Could you check a few things on this model? Use its own coordinates, in mm. Round coordinates to 2 decimals unless told otherwise and drop trailing zeros. Loops run counter-clockwise (first coordinate to the right, second up) from the corner with the lowest first, then second, coordinate; pieces in that order, holes last. Notation, with made-up numbers: (7, -15) -> (14, -15) arc R20 cw to (14, -4) -> close; hole circle Ø6 at (62, 31). An arc over 180 degrees is marked (long way). Write each question's results on one line, items separated by ' | '.
from build123d import *

# Parameters (mm, degrees)
F0_R     = 12.7
F1_DEPTH = 63.5
F2_SIZE  = 5.08


# Not quite as in the source:
# - a fillet or chamfer that OpenCascade refuses, or shapes differently, is made with other operations: its cross-section is extruded or revolved along the edge and cut away or added


with BuildPart() as f1:
    # F0 (on Front) → F1 (new body)
    with BuildSketch(Plane.XZ):
        Circle(F0_R)
    extrude(amount=F1_DEPTH)

    # F2
    f2_edges = [f1.edges().sort_by_distance(p)[0] for p in [
        (-12.7, 0, 0),
    ]]
    chamfer(f2_edges, length=F2_SIZE)

    # F3: fillet of radius 12.7 on 1 edges, made by hand

    # F3_s1 → F3_t2 (revolve, cut)
    with BuildSketch(Plane.XY):
        with BuildLine():
            add(Edge.make_bspline(
                [(12.7, -50.8), (12.7, -63.5), (0, -63.5)],
                knots=[0, 0, 0, 1, 1, 1], degree=2, weights=[1, 2.3333333333, 1]))
            Line((0, -63.5), (12.7, -63.5))
            Line((12.7, -63.5), (12.7, -50.8))
        make_face()
    revolve(axis=Axis((0, -63.5, 0), (0, -1, 0)), mode=Mode.SUBTRACT)


solid = f1.part
1) I want a section at A-A, the plane y = -11. Write out the boundary of the cut face in (x, z), plus the area to 3 significant figures.
Model answer:
outline: circle Ø25.4 at (0, 0) | area: 507 mm2
2) I need wall thicknesses on line 1 (Z direction, x = -5.5, y = -37); line 2 (Z direction, x = -11.25, y = -9); line 3 (X direction, y = -11, z = -0.75). Which ranges of each line are inside material? Lowest first, please.
Model answer:
line 1: z = -11.45 to 11.45 | line 2: z = -5.89 to 5.89 | line 3: x = -12.68 to 12.68
3) I'm going to push flat-ended pins straight in: pin 1 (8 mm diameter, centred on x = -9, z = -5.5, fed in from -Y); pin 2 (10 mm diameter, centred on x = 4, z = -7.5, fed in from -Y); pin 3 (2 mm diameter, centred on y = -54.5, z = -7, fed in from +X). Where does each tip first touch, or does it pass through?
Model answer:
pin 1: stops at y = -63.21 | pin 2: stops at y = -63.44 | pin 3: stops at x = 11.12
